CAD build for the part. Positions are in the model's coordinates, mm. A direction names the side the tool comes from. Coordinates: 2 decimals unless noted, no trailing zeros. Order: outer loops, then holes, each group sorted by start corner. A loop starts at its lowest first (then second) coordinate and runs counter-clockwise, first axis right, second up. Notation, with made-up numbers: M 36.5,35 L 75.5,35 A20 ccw 75.5,68 Z; hole C 55,30.5 d10. An arc over 180 degrees is marked long. Write item = value, one per line.
Autodesk Inventor part; units mm, degrees
ref_plane "YZ Plane" through (0, 0, 0) normal (1, 0, 0) x (0, 1, 0)
ref_plane "XZ Plane" through (0, 0, 0) normal (0, 1, 0) x (-1, 0, 0)
ref_plane "XY Plane" through (0, 0, 0) normal (0, 0, 1) x (1, 0, 0)
sketch "草圖1" plane through (0, 0, 0) normal (0, 1, 0) x (-1, 0, 0)
  line L0 (17.5, 12.5) -> (-17.5, 12.5)
  line L1 (-17.5, 12.5) -> (-17.5, -12.5)
  line L2 (-17.5, -12.5) -> (17.5, -12.5)
  line L3 (17.5, -12.5) -> (17.5, 12.5)
  line L4 (24.5, 0) -> (-24.5, 0)
  line L5 (0, -17.5) -> (0, 17.5)
  circle A0 centre (0, 9) radius 1.5
  line L6 (11.5, 0) -> (-11.5, 0)
  line L7 (-11.5, 0) -> (-11.5, 6)
  line L8 (-11.5, 6) -> (11.5, 6)
  line L9 (11.5, 6) -> (11.5, 0)
  line L10 (-11.5, 0) -> (-13.5, 0)
  line L11 (-13.5, 0) -> (-13.5, 2.5)
  line L12 (-13.5, 2.5) -> (-11.5, 2.5)
  line L13 (-11.5, 2.5) -> (-11.5, 0)
  circle A1 centre (0, -9) radius 1.5
  line L14 (-11.5, 0) -> (-11.5, -6)
  line L15 (-11.5, -6) -> (11.5, -6)
  line L16 (11.5, -6) -> (11.5, 0)
  line L17 (-13.5, 0) -> (-13.5, -2.5)
  line L18 (-13.5, -2.5) -> (-11.5, -2.5)
  line L19 (-11.5, -2.5) -> (-11.5, 0)
  dimension "d103" = 25
  dimension "d104" = 35
  dimension "d105" = 17.5
  dimension "d106" = 12.5
  dimension "d107" = 3
  dimension "d109" = 6
  dimension "d110" = 6
  dimension "d111" = 23
  dimension "d112" = 2
  dimension "d113" = 2.5
  dimension "d115" = 18
extrude "擠出2" add sketch "草圖1" along normal mid plane 3 contours L3 L4 L9 L8 L5 A0 L0 | L5 A0 L8 L7 L12 L11 L4 L1 L0 | L3 L2 L5 A1 L15 L16 L4 | L4 L17 L18 L14 L15 L5 A1 L2 L1
fillet "圓角2" radius 3 4 edges at (-17.5, 0, 12.5) (17.5, 0, 12.5) (17.5, 0, -12.5) (-17.5, 0, -12.5)
properties part number "板子4"
(1) Slice it at C-C, the plane y = -0.6. Write the cut outline in (x, z).
Evaluation:
outline = M -17.5,-9.5 A3 ccw -14.5,-12.5 L 14.5,-12.5 A3 ccw 17.5,-9.5 L 17.5,9.5 A3 ccw 14.5,12.5 L -14.5,12.5 A3 ccw -17.5,9.5 Z; hole M -11.5,-6 L 11.5,-6 L 11.5,-2.5 L 13.5,-2.5 L 13.5,2.5 L 11.5,2.5 L 11.5,6 L -11.5,6 Z; hole C 0,-9 d3; hole C 0,9 d3
(2) Pull direction Z, two halves, no side cores. Call faces 3 (the face through (0, 0, 12.5)), 4 (the face through (11.5, 0, 4)), 5 (the face through (4, 1.5, 9)): +Z half, -Z half, draft (parallel to the pull), parting line (faces both ways), or undercut.
Evaluation:
face_3 = +Z half
face_4 = undercut
face_5 = draft
(3) Pin check, flat tip, straight feed: pin 1 Ø10 at (x, z) = (3.5, -2) entering from -Y. Stop position of the tip, or through.
Evaluation:
pin_1 = -1.5
(4) Slice it at B-B, the plane x = -6.5. Write the cut outline in (y, z).
Evaluation:
outline = M -1.5,-12.5 L 1.5,-12.5 L 1.5,-6 L -1.5,-6 Z; M -1.5,6 L 1.5,6 L 1.5,12.5 L -1.5,12.5 Z
(5) Slice it at A-A, the plane z = 5. Write the cut outline in (x, y).
Evaluation:
outline = M -17.5,-1.5 L -11.5,-1.5 L -11.5,1.5 L -17.5,1.5 Z; M 11.5,-1.5 L 17.5,-1.5 L 17.5,1.5 L 11.5,1.5 Z
(6) Slice it at D-D, the plane x = 0. Write the cut outline in (y, z).
Evaluation:
outline = M -1.5,-12.5 L 1.5,-12.5 L 1.5,-10.5 L -1.5,-10.5 Z; M -1.5,-7.5 L 1.5,-7.5 L 1.5,-6 L -1.5,-6 Z; M -1.5,6 L 1.5,6 L 1.5,7.5 L -1.5,7.5 Z; M -1.5,10.5 L 1.5,10.5 L 1.5,12.5 L -1.5,12.5 Z
(7) Tool access for faces 1 (the face through (0, 0, -6)), 2 (the face through (-16.64, 0.02, 11.6)): list every direction of +Z, -Z, +X, -X, +Y, -Y with a clear straight run to the whole face (end or side of a thin tool).
Evaluation:
face_1 = +Y, -Y
face_2 = +Z, -X, +Y, -Y
(8) Wall check: line 1 (Z direction, x = 0, y = -0.5); line 2 (X direction, y = 0.9, z = 3.5); line 3 (X direction, y = -0.1, z = 9). Give the ranges that are in metal, low to high. Write a range as from..to.
Evaluation:
line_1 = -12.5..-10.5, -7.5..-6, 6..7.5, 10.5..12.5
line_2 = -17.5..-11.5, 11.5..17.5
line_3 = -17.5..-1.5, 1.5..17.5
